For this review, take the finished solid that the model builds, in its own axes (mm). A direction names the side the tool comes from. Coordinates: 2 decimals unless noted, no trailing zeros. Loops run counter-clockwise (first coordinate to the right, second up) from the corner with the lowest first, then second, coordinate; pieces in that order, holes last. Notation, with made-up numbers: M 58.5,26 L 99.5,26 A15 cw 99.5,36 Z; hole C 60.5,18.25 d2. An arc over 180 degrees is marked long. Answer as a JSON object with one key per item and string values. Group by question number.
Item 1: Add section D-D (x = 26). State the section outline as (y, z) points.
Item 2: Add section C-C (z = 0). State the section outline as (x, y) points.
Item 3: Mouldability with a two-part tool opening along X and no side actions: class faces 4 (the face through (3.124, -13, 16)), 5 (the face through (65, 1.778, -7)), 6 (the face through (60, 0, -9.906)) as +X half, -X half, draft (parallel to the pull), parting line (faces both ways), or undercut.
Item 4: Wall thickness on L1, parallel to Y at x = 5, z = 0; L2, parallel to X at y = -1.5, z = -9.5; L3, parallel to X at y = 20, z = -14: over which ranges is each line inside the solid? List them lowest first. Write a range as from..to.
Item 5: Add section B-B (x = 8). State the section outline as (y, z) points.
Item 6: Tool access review of faces 1 (the face through (63, 4.572, -7)), 2 (the face through (59, -7, -4.826)), 3 (the face through (12.7, 0, 0)): name each direction out of +Z, -Z, +X, -X, +Y, -Y from which nothing blocks a thin tool from reaching the whole face with its end or side.
Item 7: Insertion check: pin 1 (4.5 mm diameter, centred on y = -14.5, z = -14.5, fed in from +X); pin 2 (8 mm diameter, centred on x = 39, y = 13, fed in from -Z); pin 3 (1.7 mm diameter, centred on x = 63.4, z = 6.73, fed in from -Y). Each pin has a flat end and moves straight along its axis. Give the tip position at first contact, or say it passes through.
Item 8: Add section A-A (y = 0). State the section outline as (x, z) points, then the cut area to 3 significant figures.
from build123d import *

# Parameters (mm, degrees)
SKETCH1_R                                     = 25.019
BOSS_EXTRUDE1_DEPTH                           = 5.969
SKETCH2_R                                     = 14.9733
BOSS_EXTRUDE2_DEPTH                           = 38.9128
SKETCH3_W                                     = 19.812
SKETCH3_H                                     = 19.304
BOSS_EXTRUDE3_DEPTH                           = 29.9466
CBORE_FOR_4_SOCKET_HEAD_CAP_SCREW1_AT_2_COUNT = 2
CBORE_FOR_4_SOCKET_HEAD_CAP_SCREW1_AT_2_PITCH = 29.21
CBORE_FOR_4_SOCKET_HEAD_CAP_SCREW1_AT_3_COUNT = 2
CBORE_FOR_4_SOCKET_HEAD_CAP_SCREW1_AT_3_PITCH = 29.21
CBORE_FOR_4_SOCKET_HEAD_CAP_SCREW1_AT_4_COUNT = 2
CBORE_FOR_4_SOCKET_HEAD_CAP_SCREW1_AT_4_PITCH = 41.309178157
SKETCH6_R                                     = 1.4224
SKETCH6_W                                     = 7.112
SKETCH6_H                                     = 3.556
CUT_EXTRUDE1_DEPTH                            = 5.08
SKETCH7_R                                     = 1.4224
SKETCH7_W                                     = 7.112
SKETCH7_H                                     = 3.556
CUT_EXTRUDE2_DEPTH                            = 5.08
SKETCH8_R                                     = 4.73075
CUT_EXTRUDE3_DEPTH                            = 12.7


with BuildPart() as part:
    # Sketch1 → Boss-Extrude1 (new body)
    with BuildSketch(Plane(origin=(0, 0, 0), x_dir=(0, 0, -1), z_dir=(1, 0, 0))):
        Circle(SKETCH1_R)
    extrude(amount=BOSS_EXTRUDE1_DEPTH)

    # Sketch2 → Boss-Extrude2 (add)
    with BuildSketch(Plane(origin=(5.969, 0, 0), x_dir=(0, 0, -1), z_dir=(1, 0, 0))):
        Circle(SKETCH2_R)
    extrude(amount=BOSS_EXTRUDE2_DEPTH)

    # Sketch3 → Boss-Extrude3 (add)
    with BuildSketch(Plane(origin=(44.8818, 0, 0), x_dir=(0, 0, -1), z_dir=(1, 0, 0))):
        Rectangle(SKETCH3_W, SKETCH3_H)
    extrude(amount=BOSS_EXTRUDE3_DEPTH)

    # Sketch4 → CBORE for #4 Socket Head Cap Screw1 (revolve, cut)
    with BuildSketch(Plane(origin=(5.969, 14.605, -14.605), x_dir=(0, 0, -1), z_dir=(0, 1, 0))):
        Polygon((0, 0), (0, 5.969), (1.63195, 5.969), (1.63195, 2.8448), (2.77876, 2.8448), (2.77876, 1.22936), (4.00812, 0), align=None)
    cbore_for_4_socket_head_cap_screw1 = revolve(axis=Axis((12.319, 14.605, -14.605), (-1, 0, 0)), mode=Mode.SUBTRACT)

    # CBORE for #4 Socket Head Cap Screw1 at 2: CBORE for #4 Socket Head Cap Screw1 ×2
    with Locations(*[(0, 0, i * CBORE_FOR_4_SOCKET_HEAD_CAP_SCREW1_AT_2_PITCH) for i in range(1, CBORE_FOR_4_SOCKET_HEAD_CAP_SCREW1_AT_2_COUNT)]):
        add(cbore_for_4_socket_head_cap_screw1, mode=Mode.SUBTRACT)

    # CBORE for #4 Socket Head Cap Screw1 at 3: CBORE for #4 Socket Head Cap Screw1 ×2
    with Locations(*[(0, -i * CBORE_FOR_4_SOCKET_HEAD_CAP_SCREW1_AT_3_PITCH, 0) for i in range(1, CBORE_FOR_4_SOCKET_HEAD_CAP_SCREW1_AT_3_COUNT)]):
        add(cbore_for_4_socket_head_cap_screw1, mode=Mode.SUBTRACT)

    # CBORE for #4 Socket Head Cap Screw1 at 4: CBORE for #4 Socket Head Cap Screw1 ×2
    with Locations(*[Vector(0, -0.707106781, 0.707106781) * (i * CBORE_FOR_4_SOCKET_HEAD_CAP_SCREW1_AT_4_PITCH) for i in range(1, CBORE_FOR_4_SOCKET_HEAD_CAP_SCREW1_AT_4_COUNT)]):
        add(cbore_for_4_socket_head_cap_screw1, mode=Mode.SUBTRACT)

    # Sketch6 → Cut-Extrude1 (cut)
    with BuildSketch(Plane(origin=(0, 9.652, 0), x_dir=(1, 0, 0), z_dir=(0, 1, 0))):
        with Locations((63.3984, 6.731)):
            Circle(SKETCH6_R)
        with Locations((50.6984, 6.731)):
            Circle(SKETCH6_R)
        with Locations((50.6984, -6.731)):
            Circle(SKETCH6_R)
        with Locations((63.3984, -6.731)):
            Circle(SKETCH6_R)
        with Locations((57.0484, 0)):
            Rectangle(SKETCH6_W, SKETCH6_H)
    extrude(amount=-CUT_EXTRUDE1_DEPTH, mode=Mode.SUBTRACT)

    # Sketch7 → Cut-Extrude2 (cut)
    with BuildSketch(Plane(origin=(0, 0, -9.906), x_dir=(-1, 0, 0), z_dir=(0, 0, -1))):
        with Locations((-71.6534, 6.731)):
            Circle(SKETCH7_R)
        with Locations((-58.9534, 6.731)):
            Circle(SKETCH7_R)
        with Locations((-58.9534, -6.731)):
            Circle(SKETCH7_R)
        with Locations((-71.6534, -6.731)):
            Circle(SKETCH7_R)
        with Locations((-65.3034, 0)):
            Rectangle(SKETCH7_W, SKETCH7_H)
    extrude(amount=-CUT_EXTRUDE2_DEPTH, mode=Mode.SUBTRACT)

    # Sketch8 → Cut-Extrude3 (cut)
    with BuildSketch(Plane.ZY):
        Circle(SKETCH8_R)
    extrude(amount=-CUT_EXTRUDE3_DEPTH, mode=Mode.SUBTRACT)


solid = part.part
From the geometry:
{
 "1": {"outline": "C 0,0 d29.95"},
 "2": {"outline": "M 0,-25.02 L 5.97,-25.02 L 5.97,-14.97 L 44.88,-14.97 L 44.88,-9.65 L 74.83,-9.65 L 74.83,9.65 L 60.6,9.65 L 60.6,4.57 L 53.49,4.57 L 53.49,9.65 L 44.88,9.65 L 44.88,14.97 L 5.97,14.97 L 5.97,25.02 L 0,25.02 L 0,4.73 L 12.7,4.73 L 12.7,-4.73 L 0,-4.73 Z"},
 "3": {"face 4": "+X half", "face 5": "undercut", "face 6": "draft"},
 "4": {"L1": "y = -25.02..-4.73, 4.73..25.02", "L2": "x = 0..61.75, 68.86..74.83", "L3": "x = 0..5.97"},
 "5": {"outline": "C 0,0 d29.95; hole C 0,0 d9.46"},
 "6": {"face 1": "+Y", "face 2": "-Z", "face 3": "-X"},
 "7": {"pin 1": "stops at x = 3.12", "pin 2": "stops at z = -11.97", "pin 3": "stops at y = -9.65"},
 "8": {"outline": "M 0,-25.02 L 5.97,-25.02 L 5.97,-14.97 L 44.88,-14.97 L 44.88,-9.91 L 61.75,-9.91 L 61.75,-4.83 L 68.86,-4.83 L 68.86,-9.91 L 74.83,-9.91 L 74.83,9.91 L 44.88,9.91 L 44.88,14.97 L 5.97,14.97 L 5.97,25.02 L 0,25.02 L 0,4.73 L 12.7,4.73 L 12.7,-4.73 L 0,-4.73 Z", "area": "1,900 mm²"}
}
